Part model, mm, in its own coordinate system. Round coordinates to 2 decimals unless told otherwise and drop trailing zeros. Write each loop counter-clockwise with the first axis right and the second up, starting at its lowest first coordinate (ties: lowest second). Pieces come first, ordered by that corner, then holes.
Autodesk Inventor part; units mm, degrees
ref_plane "Work Plane1" through (2.75, 0, 0) normal (0, -1, 0) x (1, 0, 0)
ref_plane "YZ Plane" through (0, 0, 0) normal (1, 0, 0) x (0, 1, 0)
ref_plane "XZ Plane" through (0, 0, 0) normal (0, 1, 0) x (-1, 0, 0)
sketch "Skizze1" plane through (0, 0, 0) normal (0, 0, 1) x (1, 0, 0)
  line L0 (25, 6) -> (25, 0)
  line L1 (-18, 0) -> (25, 0)
  line L2 (-26.6, 0) -> (33.6, 0)
  line L3 (0, 7.2) -> (0, -1.2)
  line L4 (-18, 6) -> (-18, 0)
  line L5 (2, 6) -> (2, 0) construction
  line L6 (-26.6, 0) -> (33.6, 0)
  line L7 (-18, 6) -> (25, 6)
  dimension "d4" = 18
  dimension "d5" = 25
  dimension "d6" = 23
  dimension "d13" = 12
revolve "Körper" add sketch "Skizze1" angle 360 about axis through (-18, 0, 0) along (1, 0, 0)
thread "Gewinde1"
thread "Gewinde2"
chamfer "Fase1" distance 0.7678 distance2 0.7668 1 edges at (25, -6, 0) measured on face at (25, -3.0269, -1.5886)
chamfer "Fase2" distance 0.6776 distance2 0.7668 1 edges at (-18, -6, 0) measured on face at (10.1555, 5.9223, -0.9625)
ref_plane "Work Plane1" through (2.75, 0, 0) normal (0, -1, 0) x (1, 0, 0)
equation "\"d4\" = KOH"
equation "\"d5\" = NLG"
equation "\"d6\" = GEL"
equation "\"d13\" = GD"
equation "\"d1\" = KOH"
equation "\"d7\" = GEL + GAL"
equation "\"d10\" = -0.5 * SPD + 0.5 * GD"
equation "\"d12\" = -0.5 * SPD + 0.5 * GD"
equation "\"NLG\" = 25"
equation "\"GEL\" = 23"
equation "\"GAL\" = 0.61345 * PTC"
equation "\"SPD\" = NND - 1.2269 * PTC"
equation "\"d0\" = GD"
equation "\"GUL\" = 0.61345 * PTC"
equation "\"KOH\" = 18"
equation "\"GD\" = NND"
equation "\"BDM\" = NND"
equation "\"GUL1\" = 0.67658"
equation "\"GAL1\" = GAL"
equation "\"d80\" = -GUL - GEL"
equation "\"d86\" = -KOH + GUL1"
equation "\"PTC\" = 1.25"
equation "\"THREADDIA\" = 12"
equation "\"TOA\" = 30deg"
equation "\"NND\" = 12"
equation "\"GD1\" = THREADDIA - 1.2269 * PTC"
properties part number "UNI 5910 - M12 x 1,25 x 25" material "Steel, Mild"
Q1. Wall check: L1, parallel to Y at x = -11.5, z = 0.25; L2, parallel to Z at x = 10.5, y = -0.5; L3, parallel to Y at x = 11, z = -5. Give the ranges that are in metal, low to high.
Values follow:
L1: y = -5.99 to 5.99
L2: z = -5.98 to 5.98
L3: y = -3.32 to 3.32
Q2. Cut at A-A on x = 20. Write the cut outline in (y, z).
Values follow:
outline: circle Ø12 at (0, 0)
Q3. Drop flat-ended pins along their axis: pin 1 (3 mm diameter, centred on x = 18.5, y = 4.5, fed in from -Z); pin 2 (1 mm diameter, centred on x = 20, z = -3.5, fed in from -Y); pin 3 (2 mm diameter, centred on x = 2.5, z = 3, fed in from +Y). Give the stop position or say it passes through.
Values follow:
pin 1: stops at z = -5.2
pin 2: stops at y = -5.2
pin 3: stops at y = 5.66
